```python
from build123d import *

# Parameters (mm, degrees)
ESQUISSE1_R             = 4.25
ESQUISSE1_R_2           = 2
BOSS_EXTRU_1_DEPTH      = 1.6
ESQUISSE2_R             = 9.5
ESQUISSE2_R_2           = 4.5
BOSS_EXTRU_2_DEPTH      = 11.5
CONG_1_R                = 1
BOSS_EXTRU_3_DEPTH      = 13
ESQUISSE4_R             = 2
ENL_V_MAT_EXTRU_1_DEPTH = 19.5


with BuildPart() as part:
    # Esquisse1 → Boss.-Extru.1 (new body)
    with BuildSketch(Plane(origin=(0, 0, 0), x_dir=(1, 0, 0), z_dir=(0, 1, 0))):
        with BuildLine():
            Line((0, 11.5), (-25, 11.5))
            ThreePointArc((-25, 11.5), (-31.5, 5), (-25, -1.5))
            Line((-25, -1.5), (-16.90921754, -1.5))
            ThreePointArc((-16.90921754, -1.5), (-13.826301978, -3.956560509), (-15.532463951, -7.510159982))
            Line((-15.532463951, -7.510159982), (-17.532463951, -8.477187494))
            Line((-17.532463951, -8.477187494), (-13, -18.5))
            Line((-13, -18.5), (4.73848504, -10.478394893))
            ThreePointArc((4.73848504, -10.478394893), (11.241697854, 2.423680954), (0, 11.5))
        make_face()
        Circle(ESQUISSE1_R, mode=Mode.SUBTRACT)
        with Locations((-25, 5)):
            Circle(ESQUISSE1_R_2, mode=Mode.SUBTRACT)
    extrude(amount=BOSS_EXTRU_1_DEPTH)

    # Esquisse2 → Boss.-Extru.2 (add)
    with BuildSketch(Plane(origin=(0, 1.6, 0), x_dir=(1, 0, 0), z_dir=(0, 1, 0))):
        Circle(ESQUISSE2_R)
        Circle(ESQUISSE2_R_2, mode=Mode.SUBTRACT)
    extrude(amount=-BOSS_EXTRU_2_DEPTH)

    # Congé1
    cong_1_edges = [part.edges().sort_by_distance(p)[0] for p in [
        (-9.5, -9.9, 0),
    ]]
    fillet(cong_1_edges, radius=CONG_1_R)

    # Esquisse3 → Boss.-Extru.3 (add)
    with BuildSketch(Plane(origin=(0, 1.6, 0), x_dir=(1, 0, 0), z_dir=(0, 1, 0))):
        Polygon((-17.532463951, -8.477187494), (-13, -18.5), (-11.633703391, -17.88214048), (-16.182035998, -7.824237002), align=None)
    extrude(amount=BOSS_EXTRU_3_DEPTH)

    # Esquisse4 → Enlèv. mat.-Extru.1 (cut, through all)
    with BuildSketch(Plane.XY):
        with Locations((0, -4)):
            Circle(ESQUISSE4_R)
    extrude(amount=ENL_V_MAT_EXTRU_1_DEPTH, mode=Mode.SUBTRACT)


solid = part.part
```
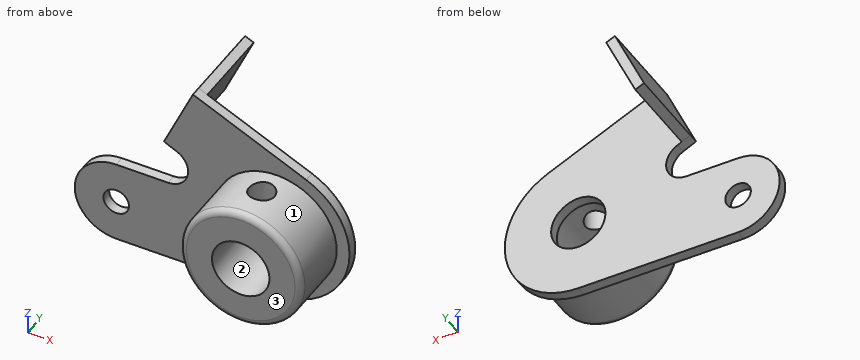
The listing builds one solid part. Answer for the finished solid, in the listing's coordinates (mm). Face numbers are marked on the shaded views. Give positions to 0.01 mm unless a question says otherwise; leave off trailing zeros. Order: outer loops, then holes, each group sorted by start corner. A loop starts at its lowest first (then second) coordinate and runs counter-clockwise, first axis right, second up. Notation, with made-up numbers: (29, 20) - (55, 20) arc R20 ccw to (55, 56) - close; hole circle Ø10 at (51.5, 37.25). An arc over 180 degrees is marked (long way). Answer in a Markdown table with one row per item. Add a question column.
Q1. The part is cut by section D-D (x = -12.5). Determine the outline of the cut face in (y, z).
Q2. The part is cut by section A-A (x = -24). Determine the outline of the cut face in (y, z), then the cut area to 3 significant figures.
Q3. The part is cut by section C-C (z = 15.5). Determine the outline of the cut face in (x, y).
Q4. For a pull along X with two mould halves and no side action, classify the marked faces 1, 2 and 3 as released by +X, released by -X, zero draft, split by the parting line, or undercut.
Q5. Find the intervals of material crossed by line 1 along Z through (x, y) = (-25, 0.55); line 2 along X through (y, z) = (-6.5, 0); line 3 along Y through (x, z) = (-6, 11.5), in increasing order. Write a range as [from, to].
Q6. The part is cut by section B-B (y = -0.75). Determine the outline of the cut face in (x, z).
Q7. Given P1, Ø10, axis at y = -7, z = -1.5, coming from the +X side; P2, Ø5, axis at y = 5.5, z = -5.5, coming from the +X side; P3, Ø5, axis at x = 0, y = -4, coming from the -Z side; P4, Ø15, axis at x = -17, z = 2.5, coming from the -Y side, each flat-ended and moving along its own axis, determine where each tip first touches the part or whether it passes through.
Determined:
| question | item | result |
|---|---|---|
| 1 | outline | (0, -11.5) - (1.6, -11.5) - (1.6, 15.97) - (14.6, 15.97) - (14.6, 18.27) - (0, 18.27) - close |
| 2 | outline | (0, -11.5) - (1.6, -11.5) - (1.6, -6.73) - (0, -6.73) - close; (0, -3.27) - (1.6, -3.27) - (1.6, 1.5) - (0, 1.5) - close |
| 2 | area | 15.3 mm² |
| 3 | outline | (-14.36, 0) - (-6.37, 0) - (-6.37, 1.6) - (-12.71, 1.6) - (-12.71, 14.6) - (-14.36, 14.6) - close |
| 4 | face 1 | split by the parting line |
| 4 | face 2 | undercut |
| 4 | face 3 | zero draft |
| 5 | line 1 | z = [-11.5, -7], [-3, 1.5] |
| 5 | line 2 | x = [-9.5, -4.5], [4.5, 9.5] |
| 5 | line 3 | y = [0, 1.6] |
| 6 | outline | circle Ø19 at (0, 0); hole circle Ø9 at (0, 0) |
| 7 | P1 | stops at x = 9.5 |
| 7 | P2 | passes through |
| 7 | P3 | stops at z = -9.5 |
| 7 | P4 | stops at y = 0 |
